Here's how the part is built. I have some questions about the finished solid (model axes, mm). A direction names the side the tool comes from. Coordinates: 2 decimals unless noted, no trailing zeros. Write each loop counter-clockwise with the first axis right and the second up, starting at its lowest first coordinate (ties: lowest second). Pieces come first, ordered by that corner, then holes.
Item 1: I want a section at D-D (y = -9.5). Please give me the cut outline in (x, z).
Item 2: If we mould it in two halves opening along Z, with no side actions, what happens to faces 6 (the face through (14, 11, 1)), 7 (the face through (17.255, -4.705, 42.038)), 8 (the face through (14, 3, 0)), 9 (the face through (17, -29, 42))? For each: pulls with the +Z half, pulls with the -Z half, needs draft (parallel to the pull), parting line crosses it, or undercut.
Item 3: I want a section at A-A (x = 25.5). Please give me the cut outline in (y, z), and give its area (3 significant figures).
Item 4: For faces 1 (the face through (17, 0, 19)), 2 (the face through (17.26, -25.57, 38.4)), 3 (the face through (33, 16, 2)), 4 (the face through (17, -2, 15)), 5 (the face through (14, 4, 1)), which set-ups out of +Z, -Z, +X, -X, +Y, -Y let a thin tool reach every point of the face, with its end or its side?
Item 5: Please list where these lines run through material, in increasing order: line 1 (Z direction, x = 33.5, y = 11.5); line 2 (Z direction, x = 13, y = 8.5); line 3 (Y direction, x = 33, z = 16).
Item 6: I'm going to push flat-ended pins straight in: P1, Ø6, axis at x = 23.5, y = 8.5, coming from the +Z side; P2, Ø7, axis at x = 19.5, z = 23, coming from the +Y side; P3, Ø2, axis at x = 5.5, y = 2, coming from the +Z side. Where does each tip first touch, or does it pass through?
Item 7: I want a section at C-C (x = 14.5). Please give me the cut outline in (y, z).
Item 8: I want a section at B-B (z = 13.5). Please give me the cut outline in (x, y), and give its area (3 significant figures).
from build123d import *

# Parameters (mm, degrees)
F1_DEPTH = 35
F2_W     = 35
F2_H     = 3
F3_DEPTH = 17
F4_W     = 10
F4_H     = 10
F5_DEPTH = 1.5
F6_SIZE  = 3
F7_R     = 5


with BuildPart() as f1:
    # F0 (on Right) → F1 (new body)
    with BuildSketch(Plane.YZ):
        with BuildLine():
            ThreePointArc((-29, 44), (-28.7071067812, 44.7071067812), (-28, 45))
            Line((-28, 45), (-16.5, 45))
            ThreePointArc((-16.5, 45), (-6.2469516728, 40.7530483272), (-2, 30.5))
            Line((-2, 30.5), (-2, 0))
            Line((-2, 0), (0, 0))
            Line((0, 0), (0, 30.5))
            ThreePointArc((0, 30.5), (-4.8327381104, 42.1672618896), (-16.5, 47))
            Line((-16.5, 47), (-31, 47))
            Line((-31, 47), (-31, 37))
            Line((-31, 37), (-25, 37))
            ThreePointArc((-25, 37), (-25.5857864376, 38.4142135624), (-27, 39))
            Line((-27, 39), (-28, 39))
            ThreePointArc((-28, 39), (-28.7071067812, 39.2928932188), (-29, 40))
            Line((-29, 40), (-29, 44))
        make_face()
    extrude(amount=F1_DEPTH)

    # F2 (on face) → F3 (join)
    with BuildSketch(Plane(origin=(0, 0, 0), x_dir=(-1, 0, 0), z_dir=(0, 1, 0))):
        with Locations((-17.5, 1.5)):
            Rectangle(F2_W, F2_H)
    extrude(amount=F3_DEPTH)

    # F4 (on face) → F5 (cut)
    with BuildSketch(Plane(origin=(0, 0, 0), x_dir=(1, 0, 0), z_dir=(0, 0, -1))):
        with Locations((17.5, -7.5)):
            Rectangle(F4_W, F4_H)
    extrude(amount=-F5_DEPTH, mode=Mode.SUBTRACT)

    # F6
    f6_edges = [f1.edges().sort_by_distance(p)[0] for p in [
        (22.5, 2.5, 0.75),
        (22.5, 12.5, 0.75),
        (12.5, 12.5, 0.75),
        (12.5, 2.5, 0.75),
    ]]
    chamfer(f6_edges, length=F6_SIZE)

    # F7
    f7_edges = [f1.edges().sort_by_distance(p)[0] for p in [
        (0, 17, 1.5),
        (35, 17, 1.5),
        (17.5, 0, 3),
    ]]
    fillet(f7_edges, radius=F7_R)


solid = f1.part
Answer:
1. outline: (0, 43.2) - (35, 43.2) - (35, 45.44) - (0, 45.44) - close
2. face 6: needs draft
2. face 7: pulls with the +Z half
2. face 8: pulls with the -Z half
2. face 9: undercut
3. outline: (-31, 37) - (-25, 37) arc R2 ccw to (-27, 39) - (-28, 39) arc R1 cw to (-29, 40) - (-29, 44) arc R1 cw to (-28, 45) - (-16.5, 45) arc R14.5 cw to (-2, 30.5) - (-2, 0) - (17, 0) - (17, 3) - (5, 3) arc R5 cw to (0, 8) - (0, 30.5) arc R16.5 ccw to (-16.5, 47) - (-31, 47) - close
3. area: 219 mm2
4. face 1: +Z, +X, -X, +Y
4. face 2: +X, -X
4. face 3: +Z, -Z, +X, +Y
4. face 4: -Z, +X, -X, -Y
4. face 5: -Z
5. line 1: z = 0 to 3
5. line 2: z = 1.5 to 3
5. line 3: y = -2 to 0
6. P1: stops at z = 3
6. P2: stops at y = 0
6. P3: stops at z = 5
7. outline: (-31, 37) - (-25, 37) arc R2 ccw to (-27, 39) - (-28, 39) arc R1 cw to (-29, 40) - (-29, 44) arc R1 cw to (-28, 45) - (-16.5, 45) arc R14.5 cw to (-2, 30.5) - (-2, 0) - (3.5, 0) - (3.5, 1.5) - (11.5, 1.5) - (11.5, 0) - (17, 0) - (17, 3) - (5, 3) arc R5 cw to (0, 8) - (0, 30.5) arc R16.5 ccw to (-16.5, 47) - (-31, 47) - close
8. outline: (0, -2) - (35, -2) - (35, 0) - (0, 0) - close
8. area: 70.0 mm2
